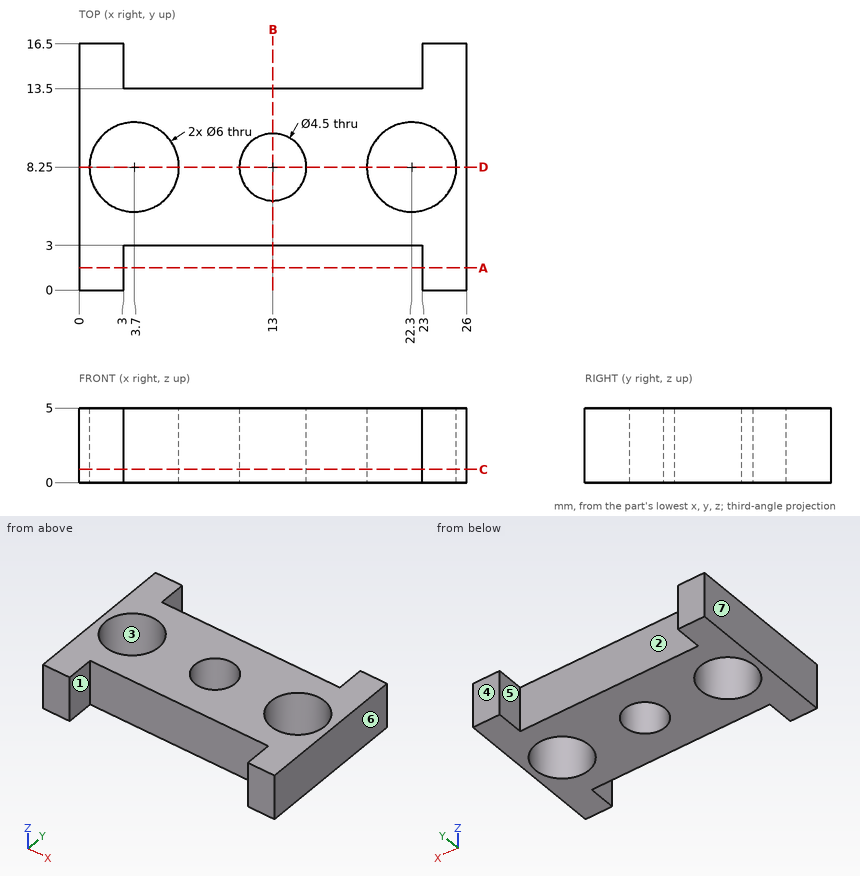
The figure shows three views and two pictorial views of one solid part (mm, origin at its lowest corner). Answer the questions. A direction names the side the tool comes from. Give positions to 0.01 mm unless a question says otherwise; leave off trailing zeros. Write each loop counter-clockwise with the first axis right and the second up, starting at its lowest first coordinate (ties: lowest second). Pieces come first, ordered by that corner, then holes. Notation, with made-up numbers: (-32, -11.75) -> (-16, -11.75) arc R28 cw to (-16, 12.25) -> close; hole circle Ø6 at (81, 21). An arc over 180 degrees is marked (long way). Answer as a JSON object with one key per item and string values.
1) A tool of negligible diameter and unlimited length cuts with its end or side. For the marked faces 1, 2 and 3, from which of +Z, -Z, +X, -X, +Y, -Y can it reach the whole face along a straight path? Write none if from no direction.
Findings below:
{"face 1": "+Z, -Z, -Y", "face 2": "+Z, -Z, +Y", "face 3": "+Z, -Z"}
2) Section D-D on y = 8.25 is taken. Write down the section's boundary in (x, z).
Findings below:
{"outline": "(0, 0) -> (0.7, 0) -> (0.7, 5) -> (0, 5) -> close; (6.7, 0) -> (10.75, 0) -> (10.75, 5) -> (6.7, 5) -> close; (15.25, 0) -> (19.3, 0) -> (19.3, 5) -> (15.25, 5) -> close; (25.3, 0) -> (26, 0) -> (26, 5) -> (25.3, 5) -> close"}
3) Straight lines are drawn through the part: probe 1 along Y at (x, z) = (3.5, 4.7); probe 2 along X at (y, z) = (13.75, 4.4); probe 3 along X at (y, z) = (7.25, 2.05). For each, find the intervals that lie inside material, in ascending order. Write a range as from..to.
Findings below:
{"probe 1": "y = 3..5.26, 11.24..13.5", "probe 2": "x = 0..3, 23..26", "probe 3": "x = 0..0.87, 6.53..10.98, 15.02..19.47, 25.13..26"}
4) Section C-C on z = 0.9 is taken. Write down the section's boundary in (x, y).
Findings below:
{"outline": "(0, 0) -> (3, 0) -> (3, 3) -> (23, 3) -> (23, 0) -> (26, 0) -> (26, 16.5) -> (23, 16.5) -> (23, 13.5) -> (3, 13.5) -> (3, 16.5) -> (0, 16.5) -> close; hole circle Ø6 at (3.7, 8.25); hole circle Ø4.5 at (13, 8.25); hole circle Ø6 at (22.3, 8.25)"}
5) Section A-A on y = 1.5 is taken. Write down the section's boundary in (x, z), then the cut area to 3 significant figures.
Findings below:
{"outline": "(0, 0) -> (3, 0) -> (3, 5) -> (0, 5) -> close; (23, 0) -> (26, 0) -> (26, 5) -> (23, 5) -> close", "area": "30.0 mm^2"}
6) A flat-ended cylindrical pin translates along its axis: pin 1 Ø1.5 at (x, z) = (9.5, 3) entering from +Y. Find the tip coordinate at first contact, or state that the pin passes through.
Findings below:
{"pin 1": "stops at y = 13.5"}
7) For a pull along X with two mould halves and no side action, classify the marked faces 4, 5, 6 and 7 as pulls with the +X half, pulls with the -X half, needs draft (parallel to the pull), parting line crosses it, or undercut.
Findings below:
{"face 4": "needs draft", "face 5": "undercut", "face 6": "pulls with the +X half", "face 7": "pulls with the -X half"}
8) Section B-B on x = 13 is taken. Write down the section's boundary in (y, z).
Findings below:
{"outline": "(3, 0) -> (6, 0) -> (6, 5) -> (3, 5) -> close; (10.5, 0) -> (13.5, 0) -> (13.5, 5) -> (10.5, 5) -> close"}
